Verification items for this drawing (mm, ordinates from the low corner). Coordinates: 2 decimals unless noted, no trailing zeros. Write each loop counter-clockwise with the first axis right and the second up, starting at its lowest first coordinate (ties: lowest second). Pieces come first, ordered by that corner, then holes.
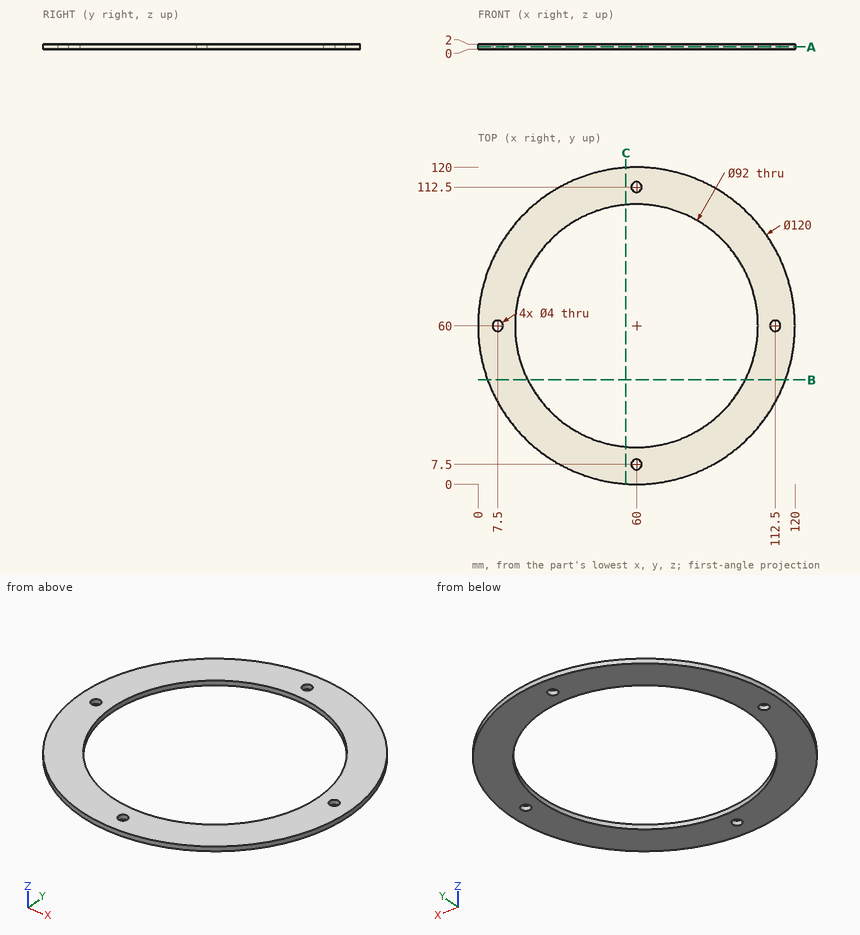
1. Sectioned sample at B-B, the plane y = 39.5. Record the boundary of the cut face in (x, z), and give its area (3 significant figures).
Computed values:
outline: (3.61, 0) - (18.82, 0) - (18.82, 2) - (3.61, 2) - close; (101.18, 0) - (116.39, 0) - (116.39, 2) - (101.18, 2) - close
area: 60.8 mm2
2. Sectioned sample at C-C, the plane x = 56. Record the boundary of the cut face in (y, z), and give its area (3 significant figures).
Computed values:
outline: (0.13, 0) - (14.17, 0) - (14.17, 2) - (0.13, 2) - close; (105.83, 0) - (119.87, 0) - (119.87, 2) - (105.83, 2) - close
area: 56.2 mm2
3. Sectioned sample at A-A, the plane z = 0.95. Record the boundary of the cut face in (x, y).
Computed values:
outline: circle Ø120 at (60, 60); hole circle Ø4 at (7.5, 60); hole circle Ø92 at (60, 60); hole circle Ø4 at (60, 7.5); hole circle Ø4 at (60, 112.5); hole circle Ø4 at (112.5, 60)
4. Thickness scan on line 1 along Y through (x, z) = (60, 0.5); line 2 along X through (y, z) = (89, 0.75); line 3 along X through (y, z) = (112.5, 1.35). Record the ranges inside material, lowest first.
Computed values:
line 1: y = 0 to 5.5, 9.5 to 14, 106 to 110.5, 114.5 to 120
line 2: x = 7.47 to 24.29, 95.71 to 112.53
line 3: x = 30.95 to 58, 62 to 89.05
